Geometry: final body of the model. Coordinates: model frame, mm. Face numbers are marked on the shaded views. A direction names the side the tool comes from. Give positions to 0.01 mm unless a question says otherwise; leave off trailing zeros. Order: outer loops, then holes, each group sorted by start corner. A loop starts at its lowest first (then second) coordinate and runs counter-clockwise, first axis right, second up. Notation, with made-up numbers: (-15, -15.75) -> (-8, -15.75) arc R38 ccw to (-8, 22.25) -> close; hole circle Ø8 at (-31.5, 77). An arc over 180 degrees is marked (long way). One line per question, with ' | ' between items. Start each with the question number.
(1) Mould query, pull axis Z, two halves, no side actions, for the marked faces 1, 2 and 3. Classes: +Z half, -Z half, draft (parallel to the pull), parting line (faces both ways), or undercut.
(2) Section C-C (x = -11.25). Return loops of the section in (y, z), then the cut area to 3 significant figures.
(3) Set-up query: the marked faces 4, 5 and 6. Return all of +Z, -Z, +X, -X, +Y, -Y with unobstructed straight access to the full face (end or side cutting, diameter ignored); none if empty.
(4) Section D-D (y = 15). Return loops of the section in (x, z).
(5) First-contact query: pin 1 Ø2 at (x, y) = (-2, 30.5) entering from -Z; pin 2 Ø8 at (y, z) = (5, -8.5) entering from -X. Flat tips, straight axial feed; report the tip coordinate or a pass-through.
(6) Section B-B (z = -5.5). Return loops of the section in (x, y), then the cut area to 3 significant figures.
(7) Section A-A (z = -16). Return loops of the section in (x, y), then the cut area to 3 significant figures.
(8) Ray query, L1, parallel to Z at x = 1.15, y = 2; L2, parallel to Z at x = -1.5, y = 22.5; L3, parallel to X at y = 40.5, z = -7.75. Return the intervals inside material, ascending.
Autodesk Inventor part; units mm, degrees
ref_plane "YZ Plane" through (0, 0, 0) normal (1, 0, 0) x (0, 1, 0)
ref_plane "XZ Plane" through (0, 0, 0) normal (0, 1, 0) x (-1, 0, 0)
ref_plane "XY Plane" through (0, 0, 0) normal (0, 0, 1) x (1, 0, 0)
sketch "スケッチ1" plane through (0, 0, 0) normal (1, 0, 0) x (0, 1, 0)
  line L0 (45, 0) -> (0, 0)
  line L1 (0, 0) -> (0, -11.5)
  line L2 (0, -11.5) -> (45, -11.5)
  line L3 (45, -11.5) -> (45, 0)
  dimension "d0" = 45
  dimension "d1" = 11.5
extrude "押し出し1" add sketch "スケッチ1" along normal blind 3
sketch "スケッチ2" plane through (3, 0, 0) normal (1, 0, 0) x (0, 0, -1)
  circle A0 centre (1.5, 43) radius 0.8
  circle A1 centre (9.4807, 43) radius 0.8
  circle A2 centre (9.5, 2) radius 0.8
  circle A3 centre (1.5, 2) radius 0.8
  circle A4 centre (5.5, 22.5) radius 0.8
  point P0 (0, 0)
extrude "押し出し2" cut sketch "スケッチ2" against normal through all
fillet "フィレット1" radius 2 2 edges at (1.5, 45, -11.5) (1.5, 0, -11.5)
sketch "スケッチ5" plane through (0, 45, 0) normal (0, 1, 0) x (1, 0, 0)
  line L0 (-5, 3) -> (-23.5, 3)
  line L1 (-23.5, 3) -> (-23.5, 16.5)
  line L2 (-23.5, 16.5) -> (-5, 16.5)
  line L3 (-5, 16.5) -> (-5, 3)
  line L4 (0, 0) -> (-26.5, 0)
  line L5 (-26.5, 0) -> (-26.5, 19.5)
  line L6 (-26.5, 19.5) -> (0, 19.5)
  line L7 (0, 19.5) -> (0, 0)
  point P0 (3, 0)
  dimension "d15" = 18.5
  dimension "d16" = 13.5
  dimension "d17" = 3
  dimension "d18" = 5
  dimension "d19" = 3
  dimension "d20" = 3
extrude "押し出し4" add sketch "スケッチ5" against normal blind 2
sketch "スケッチ6" plane through (0, 0, 0) normal (0, 0, 1) x (1, 0, 0)
  line L0 (0, 43) -> (-26.5, 43)
  line L1 (-26.5, 43) -> (0, 27.7002)
  line L2 (0, 25.5) -> (0, 40)
  line L3 (0, 43) -> (0, 0)
  dimension "d23" = 30
extrude "押し出し5" add sketch "スケッチ6" against normal up to surface (3 mm away)
sketch "スケッチ7" plane through (0, 45, -9.5) normal (1, 0, 0) x (0, 0, -1)
  line L0 (0, 0) -> (10, 0)
  arc A0 (2, -2) -> (0, 0) centre (0, -2) ccw
  line L1 (10, -2) -> (2, -2)
  line L2 (10, 0) -> (10, -2)
  line L3 (0, 0) -> (10, 0)
  point P0 (-9.5, -45)
extrude "押し出し6" cut sketch "スケッチ7" against normal blind 1
fillet "フィレット2" radius 2 3 edges at (-26.5, 44, 0) (-26.5, 44, -19.5) (-1, 44, -19.5)
sketch "スケッチ8" plane through (0, 0, 0) normal (-1, 0, 0) x (0, 0, 1)
  circle A0 centre (-1.5, 2) radius 0.8
  circle A1 centre (-9.5, 2) radius 0.8
  circle A2 centre (-5.5, 22.5) radius 0.8
  line L0 (0, 27.7002) -> (-3, 27.7002)
  line L1 (-3, 27.7002) -> (-3, 43)
  line L2 (-3, 43) -> (-8.6807, 43)
  arc A3 (-10.2807, 43) -> (-8.6807, 43) centre (-9.4807, 43) ccw
  line L3 (-10.2807, 43) -> (-11.5, 43)
  line L4 (-11.5, 2) -> (-11.5, 43)
  arc A4 (-11.5, 2) -> (-9.5, 0) centre (-9.5, 2) ccw
  line L5 (0, 0) -> (-9.5, 0)
  line L6 (0, 27.7002) -> (0, 0)
  line L7 (-3, 39.3409) -> (0, 39.3409)
  line L8 (0, 39.3409) -> (0, 27.7002)
  line L9 (0, 27.7002) -> (-3, 27.7002)
  line L10 (-3, 27.7002) -> (-3, 39.3409)
extrude "押し出し7" add sketch "スケッチ8" along normal blind 3
equation "\"d19\" = d17"
equation "\"d20\" = d17"
properties part number "button_setter"
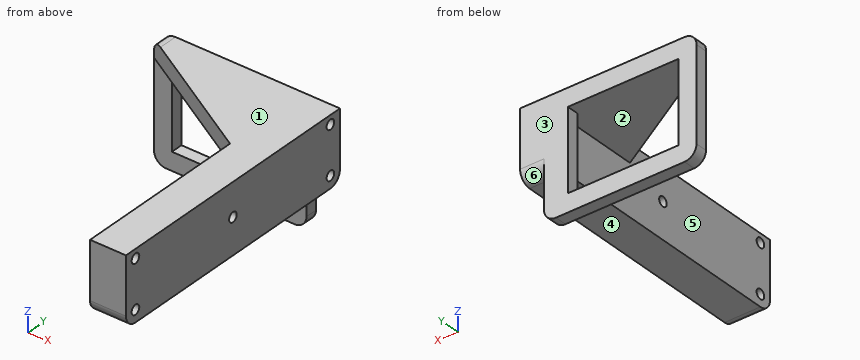
Response:
1) face 1: +Z half | face 2: undercut | face 3: draft
2) outline: (34.2, -3) -> (45, -3) -> (45, 0) -> (34.2, 0) -> close; (43, -19.5) -> (45, -19.5) -> (45, -16.5) -> (43, -16.5) -> close | area: 38.4 mm^2
3) face 4: -Z, +X, -X, -Y | face 5: -Z, -X, -Y | face 6: -Z, +X, +Y
4) outline: (-3, -11.5) -> (3, -11.5) -> (3, 0) -> (-3, 0) -> close
5) pin 1: stops at z = -11.5 | pin 2: stops at x = -3
6) outline: (-26.5, 43) -> (-23.5, 43) -> (-23.5, 45) -> (-26.5, 45) -> close; (-5, 43) -> (-3, 43) -> (-3, 23.3) -> (3, 23.3) -> (3, 45) -> (-5, 45) -> close; (-3, 0) -> (3, 0) -> (3, 21.7) -> (-3, 21.7) -> close | area: 270 mm^2
7) outline: (-26.5, 43) -> (-23.5, 43) -> (-23.5, 45) -> (-26.5, 45) -> close; (-5, 43) -> (-1, 43) -> (-1, 45) -> (-5, 45) -> close | area: 14.0 mm^2
8) L1: z = -11.5 to -10.3, -8.7 to -2.3, -0.7 to 0 | L2: z = -11.5 to -6.3, -4.7 to 0 | L3: x = -3 to 3
